Could you check a few things on this model? Use its own coordinates, in mm. Coordinates: 2 decimals unless noted, no trailing zeros. Write each loop counter-clockwise with the first axis right and the second up, starting at its lowest first coordinate (ties: lowest second). Pieces come first, ordered by that corner, then holes. Notation, with made-up numbers: M -31.75,74 L -4.75,74 A25 cw -4.75,90 Z; hole C 25,52 d6. An arc over 180 degrees is marked long. Write item = value, one per line.
```python
from build123d import *

# Parameters (mm, degrees)
SKETCH_1_W          = 19
SKETCH_1_H          = 19
SKETCH_1_W_2        = 13
SKETCH_1_H_2        = 13
EXTRUDE_1_DEPTH     = 49.33
SKETCH_2_R          = 1.65
CUT_EXTRUDE_1_DEPTH = 30
SKETCH_3_W          = 49.33
SKETCH_3_H          = 19
CUT_EXTRUDE_2_DEPTH = 16


with BuildPart() as part:
    # 草图1 → Extrude 1 (new body)
    with BuildSketch(Plane.XY):
        with Locations((6.5, 6.5)):
            Rectangle(SKETCH_1_W, SKETCH_1_H)
        with Locations((6.5, 6.5)):
            Rectangle(SKETCH_1_W_2, SKETCH_1_H_2, mode=Mode.SUBTRACT)
    extrude(amount=EXTRUDE_1_DEPTH)

    # 草图2 → 切除-拉伸1 (cut)
    with BuildSketch(Plane.ZY.offset(3)):
        with Locations((10, 6.5)):
            Circle(SKETCH_2_R)
        with Locations((39.33, 6.5)):
            Circle(SKETCH_2_R)
    extrude(amount=-CUT_EXTRUDE_1_DEPTH, mode=Mode.SUBTRACT)

    # 草图3 → 切除-拉伸2 (cut)
    with BuildSketch(Plane(origin=(16, 0, 0), x_dir=(0, 0, -1), z_dir=(1, 0, 0))):
        with Locations((-24.665, 6.5)):
            Rectangle(SKETCH_3_W, SKETCH_3_H)
    extrude(amount=-CUT_EXTRUDE_2_DEPTH, mode=Mode.SUBTRACT)


solid = part.part
```
Item 1: Imagine slicing it at A-A (z = 10). Write out the boundary of the cut face in (x, y), and give its area (3 significant figures).
Numbers:
outline = M -3,-3 L 0,-3 L 0,4.85 L -3,4.85 Z; M -3,8.15 L 0,8.15 L 0,16 L -3,16 Z
area = 47.1 mm²
Item 2: Imagine slicing it at C-C (x = -1.3). Write out the boundary of the cut face in (y, z).
Numbers:
outline = M -3,0 L 16,0 L 16,49.33 L -3,49.33 Z; hole C 6.5,10 d3.3; hole C 6.5,39.33 d3.3
Item 3: Imagine slicing it at B-B (y = 6.5). Write out the boundary of the cut face in (x, z), and give its area (3 significant figures).
Numbers:
outline = M -3,0 L 0,0 L 0,8.35 L -3,8.35 Z; M -3,11.65 L 0,11.65 L 0,37.68 L -3,37.68 Z; M -3,40.98 L 0,40.98 L 0,49.33 L -3,49.33 Z
area = 128 mm²
Item 4: If we mould it in two halves opening along Z, with no side actions, what happens to faces 1 (the face through (-2, -3, 24)), 2 (the face through (-1.521, 5.036, 10.761)), 3 (the face through (-2, 7, 0))? For each: pulls with the +Z half, pulls with the -Z half, needs draft (parallel to the pull), parting line crosses it, or undercut.
Numbers:
face_1 = needs draft
face_2 = undercut
face_3 = pulls with the -Z half
Item 5: If I drill on line 1 along Y through (x, z) = (-0.9, 39.33); line 2 along Z through (x, y) = (-0.85, 6); line 3 along Z through (x, y) = (-2.45, 6.25), over which ranges is the centre line in solid material (lowest first)?
Numbers:
line_1 = -3 to 4.85, 8.15 to 16
line_2 = 0 to 8.43, 11.57 to 37.76, 40.9 to 49.33
line_3 = 0 to 8.37, 11.63 to 37.7, 40.96 to 49.33
Item 6: I'm going to push flat-ended pins straight in: P1, Ø3, axis at y = 6.5, z = 10, coming from the +X side; P2, Ø5, axis at y = 11.5, z = 36, coming from the +X side. Where does each tip first touch, or does it pass through?
Numbers:
P1 = through
P2 = 0
